Design review of the part shown in the three views and the two pictorial views. Dimensions are in mm from the part's minimum x, y and z. Coordinates: 2 decimals unless noted, no trailing zeros. Loops run counter-clockwise (first coordinate to the right, second up) from the corner with the lowest first, then second, coordinate; pieces in that order, holes last. Notation, with made-up numbers: (3, 82.5) -> (37, 82.5) arc R7 cw to (37, 94.5) -> close; hole circle Ø10 at (31.25, 53). An arc over 180 degrees is marked (long way). Answer in a Markdown table with one row per item.
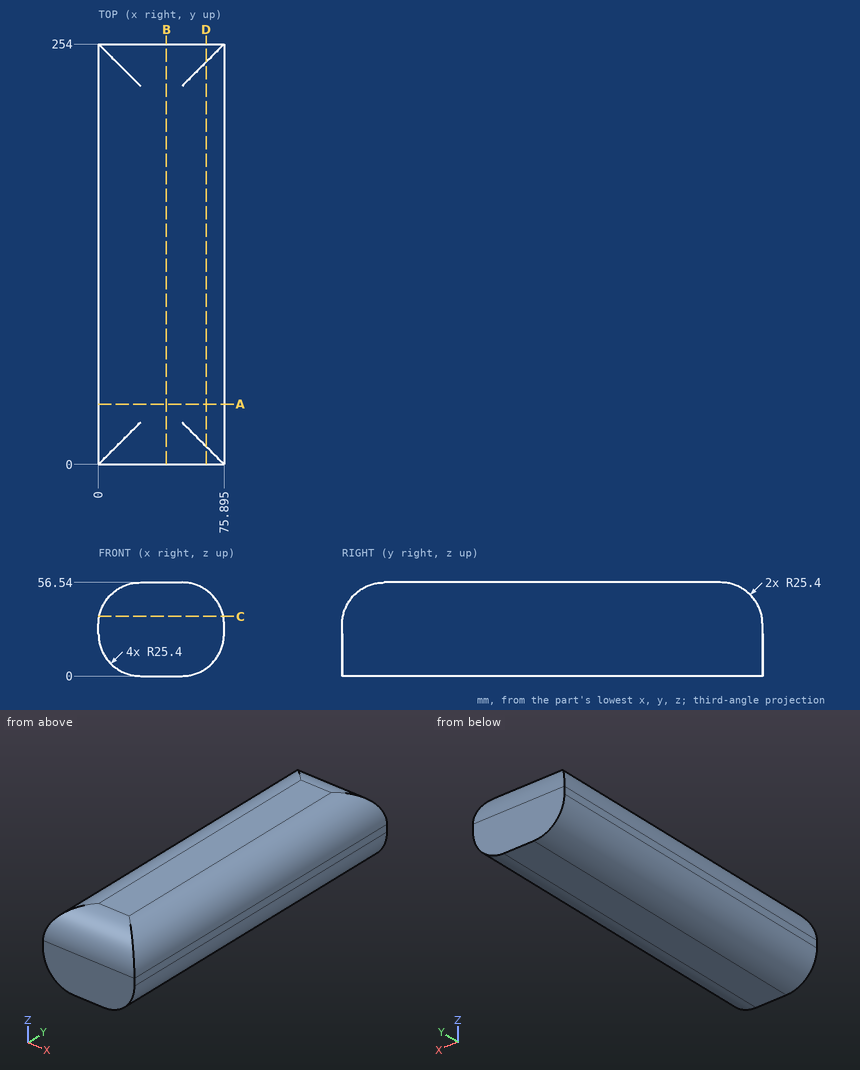
(1) For pin 1 (1.5 mm diameter, centred on x = 40.5, z = 50, fed in from -Y); pin 2 (1 mm diameter, centred on y = 207, z = 47, fed in from -X); pin 3 (10 mm diameter, centred on y = 122, z = 10.5, fed in from +X), all flat-tipped, find the tip position at first contact; note any pin that passes through.
Evaluation:
| item | result |
|---|---|
| pin 1 | stops at y = 7.59 |
| pin 2 | stops at x = 5.17 |
| pin 3 | stops at x = 73.89 |
(2) To check wall thickness, follow probe 1 along Y at (x, z) = (40, 31.5); probe 2 along X at (y, z) = (77.5, 11) (1 decimal); probe 3 along X at (y, z) = (177.5, 42). State the ranges of each line that lie inside material, in increasing order.
Evaluation:
| item | result |
|---|---|
| probe 1 | y = 0 to 254 |
| probe 2 | x = 4.5 to 71.4 |
| probe 3 | x = 2.44 to 73.46 |
(3) Take a section at D-D on x = 65. Give the boundary of the cut face in (y, z) (1 decimal).
Evaluation:
| item | result |
|---|---|
| outline | (0, 4.5) -> (254, 4.5) -> (254, 31.1) arc R25.4 ccw to (243.1, 52) -> (10.9, 52) arc R25.4 ccw to (0, 31.1) -> close |
(4) Take a section at B-B on x = 41. Give the boundary of the cut face in (y, z).
Evaluation:
| item | result |
|---|---|
| outline | (0, 0) -> (254, 0) -> (254, 31.14) arc R25.4 ccw to (228.6, 56.54) -> (25.4, 56.54) arc R25.4 ccw to (0, 31.14) -> close |
(5) Take a section at C-C on z = 36. Give the boundary of the cut face in (x, y).
Evaluation:
| item | result |
|---|---|
| outline | (0.47, 0.47) -> (75.43, 0.47) -> (75.43, 253.53) -> (0.47, 253.53) -> close |
(6) Take a section at A-A on y = 36.5. Give the boundary of the cut face in (x, z) (1 decimal).
Evaluation:
| item | result |
|---|---|
| outline | (0, 25.4) arc R25.4 ccw to (25.4, 0) -> (50.5, 0) arc R25.4 ccw to (75.9, 25.4) -> (75.9, 31.1) arc R25.4 ccw to (50.5, 56.5) -> (25.4, 56.5) arc R25.4 ccw to (0, 31.1) -> close |
